Work out the finished part from the listing and answer in its coordinate system (mm). A direction names the side the tool comes from. Coordinates: 2 decimals unless noted, no trailing zeros. Write each loop counter-clockwise with the first axis right and the second up, starting at its lowest first coordinate (ties: lowest second). Pieces come first, ordered by that corner, then holes. Notation, with made-up numbers: (48.25, -14) - (87.25, -14) arc R30 cw to (87.25, 9) - close; hole circle Ø6 at (28, 63.5). An arc over 180 degrees is marked (long way). Answer as a JSON object with one key per item and string values. Group by question number.
from build123d import *


with BuildPart() as part:
    # Sketch1 → Revolve1 (revolve)
    with BuildSketch(Plane.XY):
        with BuildLine():
            Line((18.706441928, 44.45), (0, 44.45))
            Line((0, 44.45), (0, 41.275))
            Line((0, 41.275), (12.7, 41.275))
            Line((12.7, 41.275), (12.7, 38.1))
            ThreePointArc((12.7, 38.1), (16.518963654, 37.512205275), (19.984420742, 35.803230962))
            Line((19.984420742, 35.803230962), (51.37392791, 13.824061423))
            ThreePointArc((51.37392791, 13.824061423), (53.453202163, 12.798676835), (55.744580355, 12.446))
            ThreePointArc((55.744580355, 12.446), (56.076116883, 12.467730052), (56.40198073, 12.532548401))
            Line((56.40198073, 12.532548401), (58.922800414, 13.208))
            Line((58.922800414, 13.208), (58.922800414, 19.558))
            Line((58.922800414, 19.558), (54.255902112, 19.558))
            Line((54.255902112, 19.558), (18.706441928, 44.45))
        make_face()
    revolve(axis=Axis((0, 0, 0), (1, 0, 0)))


solid = part.part
Q1. A tool of negligible diameter and unlimited length cuts with its end or side. For faces 1 (the face through (12.7, 12, -36.5)), 2 (the face through (56.6, 12, 3.8)), from which of +Z, -Z, +X, -X, +Y, -Y can it reach the whole face along a straight path? Write none if from no direction.
Q2. Section D-D on x = 36 is taken. Determine the outline of the cut face in (y, z).
Q3. Section C-C on x = 11 is taken. Determine the outline of the cut face in (y, z) (3 decimals), plus the area to 3 significant figures.
Q4. Section A-A on z = 0 is taken. Determine the outline of the cut face in (x, y) (3 decimals), plus the area to 3 significant figures.
Q5. For a pull along Y with two mould halves and no side action, classify faces 3 (the face through (6.439, -8.948, -40.293)), 4 (the face through (56.6, -4.2, -19.1)), 5 (the face through (0, 29.4, -29.4)) as +Y half, -Y half, draft (parallel to the pull), parting line (faces both ways), or undercut.
Q6. Flat-ended cylindrical pins translate along their axes: pin 1 Ø10 at (y, z) = (-8.5, 33.5) entering from +X; pin 2 Ø10 at (x, y) = (15.5, 33.5) entering from +Z; pin 3 Ø6 at (x, z) = (6, -5.5) entering from +Y. Find the tip coordinate at first contact, or state that the pin passes through.
Q7. Consider L1, parallel to Z at x = 5.25, y = 0 (3 decimals); L2, parallel to Y at x = 10, z = 15. Determine where each line is inside the solid, lowest interval first. Write a range as from..to.
Numbers:
{
 "1": {"face 1": "-X", "face 2": "+X"},
 "2": {"outline": "circle Ø64.68 at (0, 0); hole circle Ø49.18 at (0, 0)"},
 "3": {"outline": "circle Ø88.9 at (0, 0); hole circle Ø82.55 at (0, 0)", "area": "855 mm²"},
 "4": {"outline": "(0, -44.45) - (18.706, -44.45) - (54.256, -19.558) - (58.923, -19.558) - (58.923, -13.208) - (56.402, -12.533) arc R2.54 ccw to (55.745, -12.446) arc R7.62 ccw to (51.374, -13.824) - (19.984, -35.803) arc R12.7 cw to (12.7, -38.1) - (12.7, -41.275) - (0, -41.275) - close; (0, 41.275) - (12.7, 41.275) - (12.7, 38.1) arc R12.7 cw to (19.984, 35.803) - (51.374, 13.824) arc R7.62 ccw to (55.745, 12.446) arc R2.54 ccw to (56.402, 12.533) - (58.923, 13.208) - (58.923, 19.558) - (54.256, 19.558) - (18.706, 44.45) - (0, 44.45) - close", "area": "777 mm²"},
 "5": {"face 3": "undercut", "face 4": "parting line", "face 5": "draft"},
 "6": {"pin 1": "stops at x = 39.97", "pin 2": "stops at z = 34.11", "pin 3": "stops at y = 44.38"},
 "7": {"L1": "z = -44.45..-41.275, 41.275..44.45", "L2": "y = -41.84..-38.45, 38.45..41.84"}
}
